from build123d import *

# Parameters (mm, degrees)
SKETCH_2_W          = 40
SKETCH_2_H          = 40
EXTRUDE_1_DEPTH     = 10
SKETCH_3_W          = 50
SKETCH_3_H          = 16
CUT_EXTRUDE_1_DEPTH = 6.1
M2X0_4_1_D          = 1.6
M2X0_4_1_DEPTH      = 10
M2X0_4_1_TIP        = 0.480688495
SKETCH_13_W         = 10
SKETCH_13_H         = 5
EXTRUDE_5_DEPTH     = 25
M3X0_5_2_D          = 2.5
M3X0_5_2_DEPTH      = 8.5
M3X0_5_2_TIP        = 0.751075774


with BuildPart() as part:
    # ｽｹｯﾁ2 → ﾎﾞｽ - 押し出し1 (new body)
    with BuildSketch(Plane.XY):
        Rectangle(SKETCH_2_W, SKETCH_2_H)
    extrude_1 = extrude(amount=EXTRUDE_1_DEPTH)

    # ｽｹｯﾁ3 → ｶｯﾄ - 押し出し1 (cut)
    with BuildSketch(Plane.XY):
        with Locations((-13.5, 12)):
            Rectangle(SKETCH_3_W, SKETCH_3_H)
    cut_extrude_1 = extrude(amount=CUT_EXTRUDE_1_DEPTH, mode=Mode.SUBTRACT)

    # ﾐﾗｰ1: ﾎﾞｽ - 押し出し1, ｶｯﾄ - 押し出し1 across plane
    add(extrude_1.mirror(Plane.XY))
    add(cut_extrude_1.mirror(Plane.XY), mode=Mode.SUBTRACT)

    # M2x0.4 ねじ穴1
    with Locations(Plane(origin=(0, 20, 0), x_dir=(1, 0, 0), z_dir=(0, 1, 0))):
        with Locations((13.9, 0), (-13.9, 0)):
            Hole(M2X0_4_1_D / 2, depth=M2X0_4_1_DEPTH)
            with Locations((0, 0, -(M2X0_4_1_DEPTH + M2X0_4_1_TIP / 2))):  # 118° drill point
                Cone(0, M2X0_4_1_D / 2, M2X0_4_1_TIP, mode=Mode.SUBTRACT)

    # ｽｹｯﾁ13 → ﾎﾞｽ - 押し出し5 (add)
    with BuildSketch(Plane.XY.offset(10)):
        with Locations((3, -10.5)):
            Rectangle(SKETCH_13_W, SKETCH_13_H)
    extrude(amount=EXTRUDE_5_DEPTH)

    # M3x0.5 ねじ穴2
    with Locations(Plane(origin=(0, -13, 0), x_dir=(-1, 0, 0), z_dir=(0, -1, 0))):
        with Locations((-3, -20), (-3, -30)):
            Hole(M3X0_5_2_D / 2, depth=M3X0_5_2_DEPTH)
            with Locations((0, 0, -(M3X0_5_2_DEPTH + M3X0_5_2_TIP / 2))):  # 118° drill point
                Cone(0, M3X0_5_2_D / 2, M3X0_5_2_TIP, mode=Mode.SUBTRACT)


solid = part.part
Check sheet for the modelled part. Datum: model origin and axes. Units: mm. A direction names the side the tool comes from. Round coordinates to 2 decimals unless told otherwise and drop trailing zeros. Order: outer loops, then holes, each group sorted by start corner. A loop starts at its lowest first (then second) coordinate and runs counter-clockwise, first axis right, second up.
Q1. Scan lines: L1, parallel to Z at x = 3, y = -9; L2, parallel to Z at x = 13.9, y = 16.25; L3, parallel to X at y = -9.3, z = 20. Record each from-to range of solid material in increasing order.
Filled sheet:
L1: z = -10 to 18.75, 21.25 to 28.75, 31.25 to 35
L2: z = -10 to -0.8, 0.8 to 10
L3: x = -2 to 1.75, 4.25 to 8
Q2. Depth check by flat-ended pin: P1, Ø8, axis at x = 1.5, z = 18.5, coming from the +Y side; P2, Ø3.5, axis at y = 14.5, z = 0, coming from the -X side; P3, Ø4, axis at y = -10.5, z = 27.5, coming from the +X side. Enter the tip coordinate at first touch or a pass-through.
Filled sheet:
P1: stops at y = -8
P2: stops at x = 11.5
P3: stops at x = 8
Q3. Cross-section at D-D, the plane x = 9. Enter the section's corners in (y, z), plus the area to 3 significant figures.
Filled sheet:
outline: (-20, -10) - (20, -10) - (20, -6.1) - (4, -6.1) - (4, 6.1) - (20, 6.1) - (20, 10) - (-20, 10) - close
area: 605 mm2
Q4. Draft check along X on faces 4 (the face through (20, 0, 0)), 5 (the face through (4, 20, 7)), 6 (the face through (14.03, 9.6, -0.04)), 7 (the face through (2.73, -10.46, 21.22)). Enter one of: pulls with the +X half, pulls with the -X half, needs draft (parallel to the pull), parting line crosses it, or undercut.
Filled sheet:
face 4: pulls with the +X half
face 5: needs draft
face 6: undercut
face 7: undercut
Q5. Cross-section at C-C, the plane y = -11.5. Enter the section's corners in (x, z), plus the area to 3 significant figures.
Filled sheet:
outline: (-20, -10) - (20, -10) - (20, 10) - (8, 10) - (8, 35) - (-2, 35) - (-2, 10) - (-20, 10) - close; hole circle Ø2.5 at (3, 20); hole circle Ø2.5 at (3, 30)
area: 1,040 mm2
Q6. Cross-section at B-B, the plane x = 3. Enter the section's corners in (y, z).
Filled sheet:
outline: (-20, -10) - (20, -10) - (20, -6.1) - (4, -6.1) - (4, 6.1) - (20, 6.1) - (20, 10) - (-8, 10) - (-8, 18.75) - (-13, 18.75) - (-13, 10) - (-20, 10) - close; (-13, 21.25) - (-8, 21.25) - (-8, 28.75) - (-13, 28.75) - close; (-13, 31.25) - (-8, 31.25) - (-8, 35) - (-13, 35) - close
Q7. Cross-section at A-A, the plane z = 30. Enter the section's corners in (x, y).
Filled sheet:
outline: (-2, -13) - (1.75, -13) - (1.75, -8) - (-2, -8) - close; (4.25, -13) - (8, -13) - (8, -8) - (4.25, -8) - close
Q8. Set-up check for faces 1 (the face through (14.49, 14.93, -0.54)), 2 (the face through (-4, 12, 6.1)), 3 (the face through (3, -8, 22)): record each of +Z, -Z, +X, -X, +Y, -Y from which the full face is reachable in a straight line by a thin tool's end or side.
Filled sheet:
face 1: +Y
face 2: -X, +Y
face 3: +Z, +X, -X, +Y
